Part print with two shaded views. Sizes in mm from the minimum x, y, z corner. A direction names the side the tool comes from. Round coordinates to 2 decimals unless told otherwise and drop trailing zeros. Write each loop counter-clockwise with the first axis right and the second up, starting at its lowest first coordinate (ties: lowest second). Pieces come first, ordered by that corner, then holes. Notation, with made-up numbers: (20, 84) - (43, 84) arc R11 ccw to (43, 105) - close; hole circle Ø11 at (15, 30.5). An arc over 180 degrees is marked (long way). Answer as a JSON object with one key per item and string values. Group by question number.
Item 1: Flat gauge pins, fed straight in: pin 1 (2 mm diameter, centred on x = 2, z = 12.5, fed in from -Y); pin 2 (2 mm diameter, centred on y = 1.5, z = 29, fed in from +X); pin 3 (1.5 mm diameter, centred on x = 8.5, z = 39.5, fed in from -Y). Where does each tip first touch, or does it go through?
Item 2: Slice it at D-D, the plane x = 10.25. List the corners of the cut face in (y, z), then the cut area to 3 significant figures.
Item 3: Slice it at A-A, the plane x = 5.45. List the corners of the cut face in (y, z), then the cut area to 3 significant figures.
Item 4: Which spindle directions (+Z, -Z, +X, -X, +Y, -Y) get a long thin tool onto all of the face, cutting with end or side? Do the marked faces 1 and 2. Say none if no direction does.
Item 5: Probe line 1 (Y direction, x = 5.45, z = 50.8); line 2 (Z direction, x = 3, y = 8.5); line 3 (Z direction, x = 4.75, y = 4.5). List the from-to ranges inside material, lowest first. Write a range as from..to.
Item 6: Slice it at C-C, the plane z = 26. List the corners of the cut face in (x, y), then the cut area to 3 significant figures.
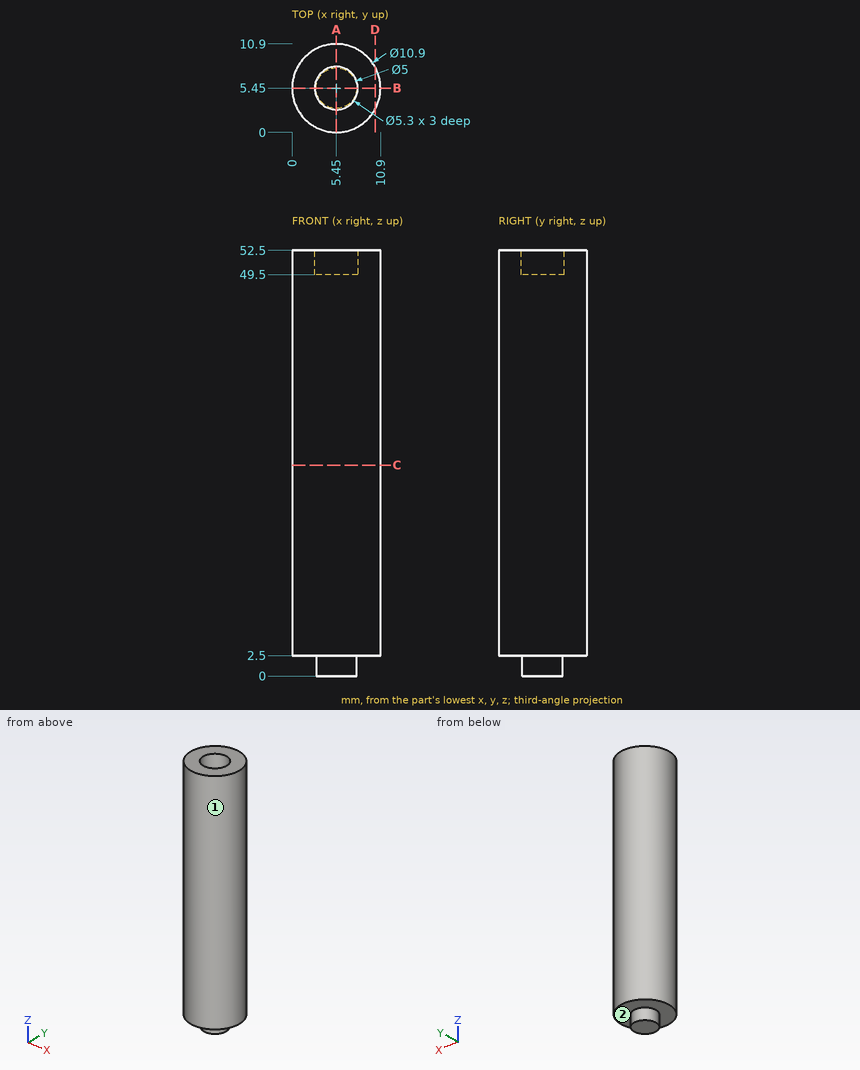
Geometry says:
{
 "1": {"pin 1": "stops at y = 0.58", "pin 2": "stops at x = 10.03", "pin 3": "stops at y = 0.51"},
 "2": {"outline": "(2.87, 2.5) - (8.03, 2.5) - (8.03, 52.5) - (2.87, 52.5) - close", "area": "258 mm^2"},
 "3": {"outline": "(0, 2.5) - (2.95, 2.5) - (2.95, 0) - (7.95, 0) - (7.95, 2.5) - (10.9, 2.5) - (10.9, 52.5) - (8.1, 52.5) - (8.1, 49.5) - (2.8, 49.5) - (2.8, 52.5) - (0, 52.5) - close", "area": "542 mm^2"},
 "4": {"face 1": "+Z, -Z", "face 2": "-Z"},
 "5": {"line 1": "y = 0..2.8, 8.1..10.9", "line 2": "z = 2.5..52.5", "line 3": "z = 0..49.5"},
 "6": {"outline": "circle Ø10.9 at (5.45, 5.45)", "area": "93.3 mm^2"}
}
